Geometry check sheet. Reference: the model listing, model coordinates, mm. Face numbers are marked on the shaded views. A direction names the side the tool comes from. Round coordinates to 2 decimals unless told otherwise and drop trailing zeros. Write each loop counter-clockwise with the first axis right and the second up, starting at its lowest first coordinate (ties: lowest second). Pieces come first, ordered by that corner, then holes.
Item 1: Cross-section at D-D (z = 18.5). Enter the section's corners in (x, y).
Item 2: Cross-section at A-A (z = 64.5). Enter the section's corners in (x, y).
Item 3: Access from +Z, -Z, +X, -X, +Y, -Y to the whole of each face (thin tool, end or side, straight path). Record for the marked faces 1, 2 and 3.
Item 4: Depth check by flat-ended pin: P1, Ø16.5, axis at y = -62, z = 52, coming from the -X side; P2, Ø4, axis at y = -25.5, z = 53.5, coming from the +X side; P3, Ø22, axis at x = 8, z = 56, coming from the -Y side. Enter the tip coordinate at first touch or a pass-through.
Item 5: Scan lines: probe 1 along Y at (x, z) = (16, 18); probe 2 along Z at (x, y) = (1, -98); probe 3 along X at (y, z) = (-52, 56). Record each from-to range of solid material in increasing order.
Item 6: Cross-section at B-B (x = 6.5). Enter the section's corners in (y, z), then the cut area to 3 significant figures.
Item 7: Draft check along X on the marked faces 4, 5 and 6. Enter one of: pulls with the +X half, pulls with the -X half, needs draft (parallel to the pull), parting line crosses it, or undercut.
Item 8: Cross-section at C-C (y = -27). Enter the section's corners in (x, z), then the cut area to 3 significant figures.
from build123d import *

# Parameters (mm, degrees)
F1_DEPTH = 160
F3_W     = 20
F3_H     = 75
F4_DEPTH = 55
F6_DEPTH = 80
F7_DEPTH = 80
F8_DEPTH = 200


with BuildPart() as f1:
    # F0 (on Front) → F1 (new body)
    with BuildSketch(Plane.XZ):
        Polygon((-21.2063081563, 25), (-16.2063081563, 70), (-21.2063081563, 70), align=None)
        Polygon((23.7936918437, 70), (-16.2063081563, 70), (-21.2063081563, 25), (-16.2063081563, 0), (23.7936918437, 0), (28.7936918437, 25), align=None)
        Polygon((28.7936918437, 70), (23.7936918437, 70), (28.7936918437, 25), align=None)
        Polygon((28.7936918437, 0), (28.7936918437, 25), (23.7936918437, 0), align=None)
        Polygon((-16.2063081563, 0), (-21.2063081563, 25), (-21.2063081563, 0), align=None)
    extrude(amount=F1_DEPTH)

    # F3 (on face) → F4 (cut)
    with BuildSketch(Plane.XY.offset(70)):
        with Locations((3.7936918437, -67.5)):
            Rectangle(F3_W, F3_H)
    extrude(amount=-F4_DEPTH, mode=Mode.SUBTRACT)

    # F5 (on face) → F6 (cut)
    with BuildSketch(Plane(origin=(-21.2063081563, 0, 0), x_dir=(0, -1, 0), z_dir=(-1, 0, 0))):
        with BuildLine():
            Line((120, 37), (120, 12))
            ThreePointArc((120, 12), (133.8212996215, 16.5538504991), (143.1985488392, 27.6818815335))
            Line((143.1985488392, 27.6818815335), (145.3737177065, 37))
            Line((145.3737177065, 37), (120, 37))
        make_face()
        with BuildLine():
            ThreePointArc((83.8675871491, 21.7687748373), (101.1727846043, 14.0695932653), (120, 12))
            Line((120, 12), (120, 37))
            Line((120, 37), (145.3737177065, 37))
            Line((145.3737177065, 37), (153.0770510435, 70))
            Line((153.0770510435, 70), (41.5276810527, 70))
            ThreePointArc((41.5276810527, 70), (44.4171997001, 68.4957364145), (46.8214808068, 66.2976555906))
            ThreePointArc((46.8214808068, 66.2976555906), (48.4316228068, 63.8555180083), (49.431870901, 61.1066824401))
            add(Edge.make_bspline(
                [(83.8675871491, 21.7687748373), (80.8791033045, 24.0777342993), (73.578379889, 29.6970945717), (57.4311562796, 47.0286131058), (51.4057960432, 57.3415797194), (49.431870901, 61.1066824401)],
                knots=[0, 0, 0, 0, 0.2722123221, 0.663175389, 0.8936579619, 0.8936579619, 0.8936579619, 0.8936579619], degree=3))
        make_face()
    extrude(amount=-F6_DEPTH, mode=Mode.SUBTRACT)

    # F2 (on face) → F7 (cut)
    with BuildSketch(Plane.YZ.offset(28.7936918437)):
        Polygon((-160, 0), (-150, 0), (-160, 70), (-160, 24.2114625871), align=None)
        Polygon((-5, 70), (0, 24.2114625871), (0, 70), align=None)
        Polygon((-5, 0), (0, 0), (0, 24.2114625871), align=None)
    extrude(amount=-F7_DEPTH, mode=Mode.SUBTRACT)

    # F0 (on Front) → F8 (cut)
    with BuildSketch(Plane.XZ):
        Polygon((28.7936918437, 70), (23.7936918437, 70), (28.7936918437, 25), align=None)
        Polygon((-21.2063081563, 25), (-16.2063081563, 70), (-21.2063081563, 70), align=None)
        Polygon((28.7936918437, 0), (28.7936918437, 25), (23.7936918437, 0), align=None)
        Polygon((-16.2063081563, 0), (-21.2063081563, 25), (-21.2063081563, 0), align=None)
    extrude(amount=F8_DEPTH, mode=Mode.SUBTRACT)


solid = f1.part
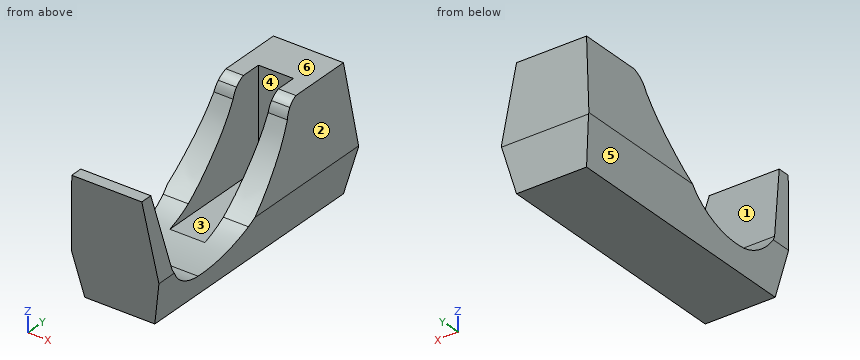
Resolved:
1. outline: (-19.91, -152.64) - (27.49, -152.64) - (27.49, -136.36) - (-19.91, -136.36) - close; (-19.91, -89.58) - (-6.21, -89.58) - (-6.21, -30) - (13.79, -30) - (13.79, -89.58) - (27.49, -89.58) - (27.49, -1.18) - (-19.91, -1.18) - close
2. outline: (-16.82, -159.21) - (24.4, -159.21) - (24.4, -151.79) - (-16.82, -151.79) - close; (-16.82, -48.08) - (-6.21, -48.08) - (-6.21, -30) - (13.79, -30) - (13.79, -48.08) - (24.4, -48.08) - (24.4, -4.4) - (-16.82, -4.4) - close
3. face 1: +Z, +X, -X
3. face 2: +Z, +X, +Y, -Y
3. face 3: +Z
4. P1: stops at x = -19.12
4. P2: stops at x = 25.85
4. P3: stops at y = -159.57
5. probe 1: y = -152.57 to -135.76, -90.6 to -1.28
5. probe 2: z = 0 to 15
5. probe 3: x = -17.76 to -6.21, 13.79 to 25.35
6. outline: (-160, 70) - (-150, 0) - (-5, 0) - (0, 24.21) - (-5, 70) - (-30, 70) - (-30, 15) - (-98.06, 15) arc R61.52 cw to (-120, 12) arc R26.69 cw to (-143.2, 27.68) - (-153.08, 70) - close
6. area: 4,230 mm2
7. face 4: undercut
7. face 5: pulls with the -X half
7. face 6: needs draft
8. outline: (-21.21, 25) - (-16.21, 0) - (23.79, 0) - (28.79, 25) - (23.79, 70) - (-16.21, 70) - close
8. area: 3,150 mm2
